from build123d import *

# Parameters (mm, degrees)
F0_R     = 41.275
F0_R_2   = 6.35
F1_DEPTH = 25.4
F2_DEPTH = 50.8
F3_R     = 2.54
F4_SIZE  = 5.08


# Not quite as in the source:
# - a feature names something its author has since deleted; it is built from what else it names


with BuildPart() as f1:
    # F0 (on Top) → F1 (new body)
    with BuildSketch(Plane.XY):
        with BuildLine():
            ThreePointArc((30.48, -40.64), (45.4369013028, -22.7184506514), (50.8, 0))
            ThreePointArc((50.8, 0), (45.4369013028, 22.7184506514), (30.48, 40.64))
            ThreePointArc((30.48, 40.64), (-50.8, 0), (30.48, -40.64))
        make_face()
        Circle(F0_R, mode=Mode.SUBTRACT)
        with BuildLine():
            ThreePointArc((71.12, 10.16), (57.8203873372, 11.3592253257), (50.8, 0))
            ThreePointArc((50.8, 0), (57.8203873372, -11.3592253257), (71.12, -10.16))
            ThreePointArc((71.12, -10.16), (74.8592253257, -5.6796126628), (76.2, 0))
            ThreePointArc((76.2, 0), (74.8592253257, 5.6796126628), (71.12, 10.16))
        make_face()
        with Locations((63.5, 0)):
            Circle(F0_R_2, mode=Mode.SUBTRACT)
        with BuildLine():
            ThreePointArc((71.12, -10.16), (57.8203873372, -11.3592253257), (50.8, 0))
            ThreePointArc((50.8, 0), (45.4369013028, -22.7184506514), (30.48, -40.64))
            Line((30.48, -40.64), (71.12, -10.16))
        make_face()
        with BuildLine():
            ThreePointArc((30.48, 40.64), (45.4369013028, 22.7184506514), (50.8, 0))
            ThreePointArc((50.8, 0), (57.8203873372, 11.3592253257), (71.12, 10.16))
            Line((71.12, 10.16), (30.48, 40.64))
        make_face()
    extrude(amount=F1_DEPTH)

    # F0 (on Top) → F2 (join)
    with BuildSketch(Plane.XY):
        with BuildLine():
            ThreePointArc((30.48, -40.64), (45.4369013028, -22.7184506514), (50.8, 0))
            ThreePointArc((50.8, 0), (45.4369013028, 22.7184506514), (30.48, 40.64))
            ThreePointArc((30.48, 40.64), (-50.8, 0), (30.48, -40.64))
        make_face()
        Circle(F0_R, mode=Mode.SUBTRACT)
    extrude(amount=F2_DEPTH)

    # F3
    f3_edges = [f1.edges().sort_by_distance(p)[0] for p in [
        (-30.48, 40.64, 50.8),
    ]]
    fillet(f3_edges, radius=F3_R)

    # F4
    f4_edges = [f1.edges().sort_by_distance(p)[0] for p in [
        (-41.275, 0, 50.8),
        (57.15, 0, 25.4),
    ]]
    chamfer(f4_edges, length=F4_SIZE)


solid = f1.part
Check sheet for the modelled part. Datum: model origin and axes. Units: mm. A direction names the side the tool comes from. Round coordinates to 2 decimals unless told otherwise and drop trailing zeros. Loops run counter-clockwise (first coordinate to the right, second up) from the corner with the lowest first, then second, coordinate; pieces in that order, holes last. Notation, with made-up numbers: (44, 79.5) -> (62, 79.5) arc R21 cw to (62, 96.5) -> close; hole circle Ø11 at (28.5, 56.5). An arc over 180 degrees is marked (long way). Put each result on its own line as item: value. Start each with the question number.
1. Section check A-A (z = 7). Enter the section's corners in (x, y) (3 decimals).
2. Access from +Z, -Z, +X, -X, +Y, -Y to the whole of each face (thin tool, end or side, straight path). Record for faces 4 (the face through (-44.26, 24.93, 23.79)), 5 (the face through (51.5, 0.2, 25.4)), 6 (the face through (41, -11, 0)).
3. Draft check along Y on faces 1 (the face through (69.594, -2.527, 20.567)), 2 (the face through (-43, 18, 50.8)), 3 (the face through (51.08, 25.19, 12.52)). Enter one of: +Y half, -Y half, draft (parallel to the pull), parting line (faces both ways), or undercut.
4. Scan lines: probe 1 along Y at (x, z) = (0, 32) (3 decimals); probe 2 along Y at (x, z) = (28, 36.5); probe 3 along X at (y, z) = (3.5, 10.5). Record each from-to range of solid material in increasing order.
5. Section check B-B (x = 63.5). Enter the section's corners in (y, z) (3 decimals).
6. Gauge pin test, flat ends, axial feed: pin 1 (8 mm diameter, centred on y = -14, z = 16, fed in from -X); pin 2 (3 mm diameter, centred on x = 21.5, z = 22.5, fed in from -Y); pin 3 (8 mm diameter, centred on y = -10, z = 26, fed in from +X). Record the tip position at first contact, or that the pin passes through.
Findings:
1. outline: (30.48, -40.64) -> (71.12, -10.16) arc R12.7 ccw to (71.12, 10.16) -> (30.48, 40.64) arc R50.8 ccw (long way) to start; hole circle Ø82.55 at (0, 0); hole circle Ø12.7 at (63.5, 0)
2. face 4: +Z
2. face 5: +Z, +X
2. face 6: -Z, +X, -X, +Y, -Y
3. face 1: undercut
3. face 2: draft
3. face 3: +Y half
4. probe 1: y = -50.8 to -41.275, 41.275 to 50.8
4. probe 2: y = -42.39 to -30.33, 30.33 to 42.39
4. probe 3: x = -50.68 to -41.13, 41.13 to 58.2, 68.8 to 75.71
5. outline: (-15.875, 0) -> (-6.35, 0) -> (-6.35, 20.32) -> (-11.43, 25.4) -> (-15.875, 25.4) -> close; (6.35, 0) -> (15.875, 0) -> (15.875, 25.4) -> (11.43, 25.4) -> (6.35, 20.32) -> close
6. pin 1: stops at x = -49.81
6. pin 2: stops at y = -46.7
6. pin 3: stops at x = 74.67
